from build123d import *

# Parameters (mm, degrees)
CHAMFER1_SIZE           = 2.54
DOME1_FACE_RADIUS       = 15.24
DOME1_HEIGHT            = 6.35
CUT_EXTRUDE5_DEPTH      = 16.24
CUT_EXTRUDE5_DEPTH_BACK = 16.24


with BuildPart() as part:
    # Sketch2 → Revolve-Thin2 (revolve)
    with BuildSketch(Plane.XY):
        Polygon((0, -85.867755946), (-6.35, -85.867755946), (-6.35, -42.687755946), (-12.7, -42.687755946), (-12.7, -40.147755946), (0, -40.147755946), (0, -37.607755946), (-15.24, -37.607755946), (-15.24, -45.227755946), (-8.89, -45.227755946), (-8.89, -88.407755946), (0, -88.407755946), align=None)
    revolve(axis=Axis((0, -25.732100586, 0), (0, -1, 0)))

    # Chamfer1
    chamfer1_edges = [part.edges().sort_by_distance(p)[0] for p in [
        (8.89, -88.407755946, 0),
    ]]
    chamfer(chamfer1_edges, length=CHAMFER1_SIZE)

    # Dome1: a dome of height H over a round flat face of radius A is a cap of a sphere of radius (A * A + H * H) / (2 * H)
    dome1_r = (DOME1_FACE_RADIUS * DOME1_FACE_RADIUS + DOME1_HEIGHT * DOME1_HEIGHT) / (2 * DOME1_HEIGHT)
    dome1_base = Plane((0, -37.607755946, 0), z_dir=(0, 1, 0))
    with Locations(dome1_base.offset(DOME1_HEIGHT - dome1_r)):
        dome1_ball = Sphere(dome1_r, mode=Mode.PRIVATE)
    add(split(dome1_ball, bisect_by=dome1_base, keep=Keep.TOP, mode=Mode.PRIVATE))

    # Sketch15 → Cut-Extrude5 (cut, two sides)
    with BuildSketch(Plane.XY) as cut_extrude5_sk:
        Polygon((63.582364053, 84.47121169), (5.21254128, -31.900338505), (2.340727282, -37.625856093), (-2.340727282, -37.625856093), (-5.21254128, -31.900338505), (-63.582364053, 84.47121169), (-63.582364053, 344.850733967), (63.582364053, 344.850733967), align=None)
    extrude(amount=CUT_EXTRUDE5_DEPTH, mode=Mode.SUBTRACT)
    extrude(cut_extrude5_sk.sketch, amount=-CUT_EXTRUDE5_DEPTH_BACK, mode=Mode.SUBTRACT)


solid = part.part
Verification items for the finished model (mm, model axes). A direction names the side the tool comes from. Coordinates: 2 decimals unless noted, no trailing zeros. Order: outer loops, then holes, each group sorted by start corner. A loop starts at its lowest first (then second) coordinate and runs counter-clockwise, first axis right, second up. Notation, with made-up numbers: (45, -15.75) -> (95, -15.75) arc R15 ccw to (95, 3.25) -> close; hole circle Ø10 at (23, 17). An arc over 180 degrees is marked (long way). Use CSV: the item, a comma, the result in double quotes. Start each with the question number.
Q1. Section check B-B, the plane z = 0. Record the cut outline in (x, y).
Q2. Section check A-A, the plane x = 0. Record the cut outline in (y, z).
Q3. Thickness scan on line 1 along Y through (x, z) = (-1.5, 5); line 2 along X through (y, z) = (-41, 0); line 3 along X through (y, z) = (-59, 0). Record the ranges inside material, lowest first.
Q4. Draft check along Z on faces 1 (the flat face through (3.478, -35.359, -0.211)), 2 (the cylindrical face through (1.38, -63.98, 6.2)), 3 (the cylindrical face through (1.93, -65.83, 8.68)), 4 (the flat face through (0, -40.148, 0)). Enter one of: +Z half, -Z half, draft (parallel to the pull), parting line (faces both ways), or undercut.
Q5. Section check D-D, the plane x = 10.5. Record the cut outline in (y, z), and give its area (3 significant figures).
Q6. Depth check by flat-ended pin: P1, Ø1, axis at y = -48.5, z = 8, coming from the +X side; P2, Ø2.5, axis at x = 0.5, z = 5.5, coming from the +Y side; P3, Ø1, axis at x = -8.5, z = -4.5, coming from the +Y side; P4, Ø1, axis at y = -67, z = 11, coming from the +X side. Enter the tip coordinate at first touch or a pass-through.
Q7. Tool access check on faces 5 (the flat face through (-7, -45.228, 7)), 6 (the flat face through (0, -88.408, 0)), 7 (the cylindrical face through (3.3, -41.47, 14.88)), 8 (the flat face through (3, -42.688, -6)), 9 (the flat face through (-3.437, -35.439, 0.211)). Record the directions out of +Z, -Z, +X, -X, +Y, -Y that give a thin tool (end or side, any length) a straight path to the whole face; none if there is none.
Q8. Section check C-C, the plane y = -64.5. Record the cut outline in (x, z), and give its area (3 significant figures).
Returned:
1,outline,"(-15.24, -45.23) -> (-8.89, -45.23) -> (-8.89, -85.87) -> (-6.35, -88.41) -> (6.35, -88.41) -> (8.89, -85.87) -> (8.89, -45.23) -> (15.24, -45.23) -> (15.24, -37.61) arc R21.46 ccw to (5.21, -31.9) -> (2.34, -37.63) -> (-2.34, -37.63) -> (-5.21, -31.9) arc R21.46 ccw to (-15.24, -37.61) -> close; hole (-12.7, -42.69) -> (-6.35, -42.69) -> (-6.35, -85.87) -> (6.35, -85.87) -> (6.35, -42.69) -> (12.7, -42.69) -> (12.7, -40.15) -> (-12.7, -40.15) -> close"
2,outline,"(-88.41, -6.35) -> (-85.87, -8.89) -> (-45.23, -8.89) -> (-45.23, -15.24) -> (-37.63, -15.24) -> (-37.63, 15.24) -> (-45.23, 15.24) -> (-45.23, 8.89) -> (-85.87, 8.89) -> (-88.41, 6.35) -> close; hole (-85.87, -6.35) -> (-42.69, -6.35) -> (-42.69, -12.7) -> (-40.15, -12.7) -> (-40.15, 12.7) -> (-42.69, 12.7) -> (-42.69, 6.35) -> (-85.87, 6.35) -> close"
3,line 1,"y = -88.41 to -85.87, -40.15 to -37.63"
3,line 2,"x = -15.24 to -12.7, 12.7 to 15.24"
3,line 3,"x = -8.89 to -6.35, 6.35 to 8.89"
4,face 1,"draft"
4,face 2,"undercut"
4,face 3,"parting line"
4,face 4,"undercut"
5,outline,"(-45.23, -11.05) -> (-37.61, -11.05) arc R18.72 ccw to (-37.61, 11.05) -> (-45.23, 11.05) -> close; hole (-42.69, -7.14) -> (-40.15, -7.14) -> (-40.15, 7.14) -> (-42.69, 7.14) -> close"
5,area,"186 mm^2"
6,P1,"stops at x = 4.77"
6,P2,"stops at y = -37.63"
6,P3,"stops at y = -33.29"
6,P4,"passes through"
7,face 5,"-Y"
7,face 6,"+Z, -Z, +X, -X, -Y"
7,face 7,"+Y, -Y"
7,face 8,"none"
7,face 9,"+Z, -Z, +Y"
8,outline,"circle Ø17.78 at (0, 0); hole circle Ø12.7 at (0, 0)"
8,area,"122 mm^2"
